Can you work these out from the model? Positions are in its coordinate system, mm. A direction names the side the tool comes from. Coordinates: 2 decimals unless noted, no trailing zeros. Write each loop counter-clockwise with the first axis right and the second up, starting at its lowest first coordinate (ties: lowest second). Pieces come first, ordered by that corner, then holes. Notation, with made-up numbers: M -14.75,-32 L 40.25,-32 A15 cw 40.25,-24 Z; hole C -24,27.5 d9. An arc over 180 degrees is marked long. Use one line per item in the form item = value. Start each with the question number.
```python
from build123d import *

# Parameters (mm, degrees)
Y_KSEKLIK_EKSTR_ZYON1_DEPTH = 4
IZIM3_R                     = 3
Y_KSEKLIK_EKSTR_ZYON2_DEPTH = 100


with BuildPart() as part:
    # Çizim2 → Yükseklik-Ekstrüzyon1 (new body)
    with BuildSketch(Plane(origin=(0, 0, 0), x_dir=(1, 0, 0), z_dir=(0, 1, 0))):
        Polygon((5.773502692, 0), (2.886751346, 5), (-2.886751346, 5), (-5.773502692, 0), (-2.886751346, -5), (2.886751346, -5), align=None)
    extrude(amount=Y_KSEKLIK_EKSTR_ZYON1_DEPTH)

    # Çizim3 → Yükseklik-Ekstrüzyon2 (add)
    with BuildSketch(Plane(origin=(0, 4, 0), x_dir=(1, 0, 0), z_dir=(0, 1, 0))):
        with Locations(Location((0, 0, 0), (0, 0, 270))):
            Circle(IZIM3_R)
    extrude(amount=Y_KSEKLIK_EKSTR_ZYON2_DEPTH)

    # Çizim4 → Kes-Döndür1 (revolve, cut)
    with BuildSketch(Plane.XY, mode=Mode.PRIVATE) as kes_d_nd_r1_sk:
        Polygon((-2.5, 103.5), (-2.5, 84.5), (-3, 84), (-5.565030224, 84), (-5.565030224, 104), (-2.5, 104), (-2.027017716, 104), align=None)
    revolve(kes_d_nd_r1_sk.sketch.rotate(Axis((0, 106.310945379, 0), (0, -1, 0)), 270), axis=Axis((0, 106.310945379, 0), (0, -1, 0)), mode=Mode.SUBTRACT)


solid = part.part
```
1) Which directions (+Z, -Z, +X, -X, +Y, -Y) give clear straight access to the entire face, cutting with the end or side of a thin tool? Please do faces 1 (the face through (2.44, 93.87, -0.54)), 2 (the face through (-4.35, 1.972, 2.465)).
2) Suppose I cut it at A-A on x = 0. Please give me the cut outline in (y, z).
3) Please list where these lines run through material, in increasing order: line 1 (X direction, y = 82.5, z = 0.25); line 2 (Y direction, x = -3.5, z = 0).
4) Will these pins go through, and if not, where does the flat tip stop? pin 1 Ø5 at (y, z) = (48, 4) entering from +X; pin 2 Ø4 at (x, y) = (0, 15) entering from +Z; pin 3 Ø1.5 at (y, z) = (19, -1.5) entering from -X.
5) Suppose I cut it at B-B on y = 75. Please give me the cut outline in (x, z).
Computed values:
q1.face_1 = +Y
q1.face_2 = +Z, -X, +Y, -Y
q2.outline = M 0,-5 L 4,-5 L 4,-3 L 84,-3 L 84.5,-2.5 L 103.5,-2.5 L 104,-2.03 L 104,2.03 L 103.5,2.5 L 84.5,2.5 L 84,3 L 4,3 L 4,5 L 0,5 Z
q3.line_1 = -2.99 to 2.99
q3.line_2 = 0 to 4
q4.pin_1 = 2.6
q4.pin_2 = 3
q4.pin_3 = -2.9
q5.outline = C 0,0 d6
